```python
from build123d import *

# Parameters (mm, degrees)
BOSS_EXTRUDE4_DEPTH = 57
FILLET4_R           = 3
SKETCH10_R          = 2.5
SKETCH10_R_2        = 19.5
CUT_EXTRUDE5_DEPTH  = 4
SKETCH11_R          = 2.5
CUT_EXTRUDE6_DEPTH  = 4


with BuildPart() as part:
    # Sketch1 → Boss-Extrude4 (new body)
    with BuildSketch(Plane(origin=(0, 0, 0), x_dir=(0, 0, -1), z_dir=(1, 0, 0))):
        Polygon((0, 0), (0, -61), (61, -61), (61, -57), (4, -57), (4, 0), align=None)
    extrude(amount=BOSS_EXTRUDE4_DEPTH)

    # Fillet4
    fillet4_edges = [part.edges().sort_by_distance(p)[0] for p in [
        (28.5, -61, 0),
    ]]
    fillet(fillet4_edges, radius=FILLET4_R)

    # Sketch10 → Cut-Extrude5 (cut)
    with BuildSketch(Plane(origin=(0, -57, 0), x_dir=(1, 0, 0), z_dir=(0, 1, 0))):
        with Locations(Location((5, 56, 0), (0, 0, 270))):
            Circle(SKETCH10_R)
        with Locations(Location((5, 9, 0), (0, 0, 270))):
            Circle(SKETCH10_R)
        with Locations(Location((52, 9, 0), (0, 0, 270))):
            Circle(SKETCH10_R)
        with Locations(Location((52, 56, 0), (0, 0, 270))):
            Circle(SKETCH10_R)
        with Locations(Location((28.5, 32.5, 0), (0, 0, 270))):
            Circle(SKETCH10_R_2)
    extrude(amount=-CUT_EXTRUDE5_DEPTH, mode=Mode.SUBTRACT)

    # Sketch11 → Cut-Extrude6 (cut)
    with BuildSketch(Plane(origin=(0, 0, -4), x_dir=(-1, 0, 0), z_dir=(0, 0, -1))):
        with Locations((-48.5, -8)):
            Circle(SKETCH11_R)
        with Locations((-48.5, -49)):
            Circle(SKETCH11_R)
        with Locations(Location((-8.5, -49, 0), (0, 0, 90))):
            Circle(SKETCH11_R)
        with Locations(Location((-8.5, -8, 0), (0, 0, 90))):
            Circle(SKETCH11_R)
    extrude(amount=-CUT_EXTRUDE6_DEPTH, mode=Mode.SUBTRACT)


solid = part.part
```
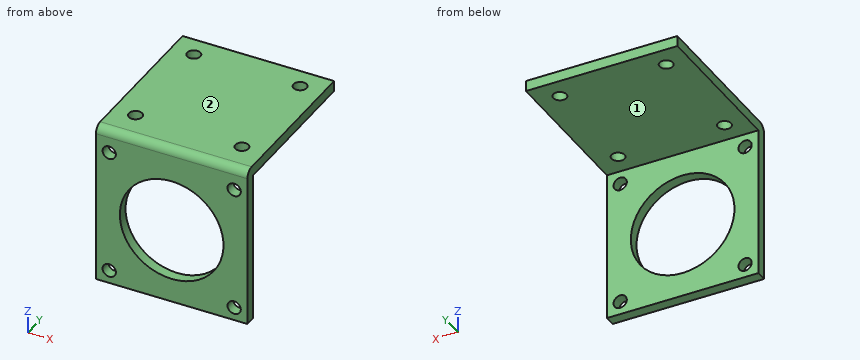
For this review, take the finished solid that the model builds, in its own axes (mm). Face numbers are marked on the shaded views. A direction names the side the tool comes from. Round coordinates to 2 decimals unless told otherwise and drop trailing zeros. Loops run counter-clockwise (first coordinate to the right, second up) from the corner with the lowest first, then second, coordinate; pieces in that order, holes last.
Q1. Add section B-B on y = -9.5. Write out the cut boundary in (x, z).
Result sheet:
outline: (0, -4) - (6.5, -4) - (6.5, 0) - (0, 0) - close; (10.5, -4) - (46.5, -4) - (46.5, 0) - (10.5, 0) - close; (50.5, -4) - (57, -4) - (57, 0) - (50.5, 0) - close
Q2. Add section D-D on z = -14.5. Write out the cut boundary in (x, y).
Result sheet:
outline: (0, -61) - (21, -61) - (21, -57) - (0, -57) - close; (36, -61) - (57, -61) - (57, -57) - (36, -57) - close
Q3. Add section C-C on x = 28.5. Write out the cut boundary in (y, z), plus the area to 3 significant figures.
Result sheet:
outline: (-61, -61) - (-57, -61) - (-57, -52) - (-61, -52) - close; (-61, -13) - (-57, -13) - (-57, -4) - (0, -4) - (0, 0) - (-58, 0) arc R3 ccw to (-61, -3) - close
area: 314 mm2
Q4. Add section A-A on z = -56. Write out the cut boundary in (x, y).
Result sheet:
outline: (0, -61) - (2.5, -61) - (2.5, -57) - (0, -57) - close; (7.5, -61) - (49.5, -61) - (49.5, -57) - (7.5, -57) - close; (54.5, -61) - (57, -61) - (57, -57) - (54.5, -57) - close
Q5. Insertion check: pin 1 Ø1 at (x, y) = (30, -20.5) entering from -Z; pin 2 Ø6 at (x, z) = (5, -56) entering from +Y. Each pin has a flat end and moves straight along its axis. Give the tip position at first contact, or say it passes through.
Result sheet:
pin 1: stops at z = -4
pin 2: stops at y = -57
Q6. Machinability: for the marked faces 1 and 2, which of the approach directions +Z, -Z, +X, -X, +Y, -Y give a long, thin tool a straight path to every point of the face, cutting with its end or side? Answer none if there is none.
Result sheet:
face 1: -Z, +X, -X, +Y
face 2: +Z, +X, -X, +Y, -Y
Q7. To check wall thickness, follow line 1 along X through (y, z) = (-58, -9); line 2 along Y through (x, z) = (38, -5); line 3 along Z through (x, y) = (31, -7.5). State the ranges of each line that lie inside material, in increasing order.
Result sheet:
line 1: x = 0 to 2.5, 7.5 to 49.5, 54.5 to 57
line 2: y = -61 to -57
line 3: z = -4 to 0
